Geometry: final body of the model. Coordinates: model frame, mm. A direction names the side the tool comes from. Coordinates: 2 decimals unless noted, no trailing zeros. Loops run counter-clockwise (first coordinate to the right, second up) from the corner with the lowest first, then second, coordinate; pieces in that order, holes last. Notation, with made-up numbers: (71.25, -16.5) - (107.25, -16.5) arc R12 ccw to (107.25, -12.5) - close; hole circle Ø7 at (61, -12). An arc over 180 degrees is marked (long way). Answer in a Markdown table with one row per item.
from build123d import *

# Parameters (mm, degrees)
ESQUISSE1_W           = 11.4
ESQUISSE1_H           = 11.4
BOSS_EXTRU_1_DEPTH    = 147.2
TROU_TARAUD_M41_D     = 3.3
TROU_TARAUD_M41_DEPTH = 11.5
TROU_TARAUD_M41_TIP   = 0.991420021
TROU_TARAUD_M42_D     = 3.3
TROU_TARAUD_M42_DEPTH = 11.5
TROU_TARAUD_M42_TIP   = 0.991420021
D_GAGEMENT_M41_D      = 4.5


with BuildPart() as part:
    # Esquisse1 → Boss.-Extru.1 (new body)
    with BuildSketch(Plane(origin=(0, 0, 0), x_dir=(1, 0, 0), z_dir=(0, 1, 0))):
        Rectangle(ESQUISSE1_W, ESQUISSE1_H)
    extrude(amount=BOSS_EXTRU_1_DEPTH)

    # Trou taraudé M41
    with Locations(Plane(origin=(0, 147.2, 0), x_dir=(-1, 0, 0), z_dir=(0, 1, 0))):
        with Locations((0, 0)):
            Hole(TROU_TARAUD_M41_D / 2, depth=TROU_TARAUD_M41_DEPTH)
            with Locations((0, 0, -(TROU_TARAUD_M41_DEPTH + TROU_TARAUD_M41_TIP / 2))):  # 118° drill point
                Cone(0, TROU_TARAUD_M41_D / 2, TROU_TARAUD_M41_TIP, mode=Mode.SUBTRACT)

    # Trou taraudé M42
    with Locations(Plane.XZ):
        with Locations((0, 0)):
            Hole(TROU_TARAUD_M42_D / 2, depth=TROU_TARAUD_M42_DEPTH)
            with Locations((0, 0, -(TROU_TARAUD_M42_DEPTH + TROU_TARAUD_M42_TIP / 2))):  # 118° drill point
                Cone(0, TROU_TARAUD_M42_D / 2, TROU_TARAUD_M42_TIP, mode=Mode.SUBTRACT)

    # Dégagement M41 (through all)
    with Locations(Plane.XY.offset(5.7)):
        with Locations((0, 128.6), (0, 73.6), (0, 18.6)):
            Hole(D_GAGEMENT_M41_D / 2)


solid = part.part
(1) Cut plane A-A on y = 18.6. Output: boundary loops of the cut face in (x, z).
Verdict:
| item | result |
|---|---|
| outline | (-5.7, -5.7) - (-2.25, -5.7) - (-2.25, 5.7) - (-5.7, 5.7) - close; (2.25, -5.7) - (5.7, -5.7) - (5.7, 5.7) - (2.25, 5.7) - close |
(2) Pull-direction query (Y, two-part tool) for faces 4 (the face through (0.488, 71.404, -0.08)), 5 (the face through (-1.3, 0, -1.3)), 6 (the face through (-3, 73, -5.7)); classes: pulls with the +Y half, pulls with the -Y half, needs draft (parallel to the pull), parting line crosses it, or undercut.
Verdict:
| item | result |
|---|---|
| face 4 | undercut |
| face 5 | pulls with the -Y half |
| face 6 | needs draft |
(3) Access query for faces 1 (the face through (-1.216, 141.37, 1.115)), 2 (the face through (5.7, 73, 0)), 3 (the face through (1.216, 5.831, 1.115)). Directions: +Z, -Z, +X, -X, +Y, -Y. A direction counts if a zero-diameter tool reaches every point of the face in a straight line with its end or side. Return the directions, or none.
Verdict:
| item | result |
|---|---|
| face 1 | +Y |
| face 2 | +Z, -Z, +X, +Y, -Y |
| face 3 | -Y |
(4) Cut plane B-B on z = 4.5. Output: boundary loops of the cut face in (x, y).
Verdict:
| item | result |
|---|---|
| outline | (-5.7, 0) - (5.7, 0) - (5.7, 147.2) - (-5.7, 147.2) - close; hole circle Ø4.5 at (0, 18.6); hole circle Ø4.5 at (0, 73.6); hole circle Ø4.5 at (0, 128.6) |
(5) Ray query, probe 1 along Y at (x, z) = (0, 1.75); probe 2 along X at (y, z) = (128.6, -1.75); probe 3 along Z at (x, y) = (0, 142.75). Return the intervals inside material, ascending.
Verdict:
| item | result |
|---|---|
| probe 1 | y = 0 to 16.35, 20.85 to 71.35, 75.85 to 126.35, 130.85 to 147.2 |
| probe 2 | x = -5.7 to -2.25, 2.25 to 5.7 |
| probe 3 | z = -5.7 to -1.65, 1.65 to 5.7 |
(6) First-contact query: pin 1 Ø1.5 at (x, z) = (0, 4.5) entering from -Y; pin 2 Ø2 at (x, z) = (0, 0) entering from -Y; pin 3 Ø2 at (x, z) = (0.5, 0) entering from +Y. Flat tips, straight axial feed; report the tip coordinate or a pass-through.
Verdict:
| item | result |
|---|---|
| pin 1 | stops at y = 0 |
| pin 2 | stops at y = 11.89 |
| pin 3 | stops at y = 135.61 |
(7) Cut plane C-C on y = 137. Output: boundary loops of the cut face in (x, z).
Verdict:
| item | result |
|---|---|
| outline | (-5.7, -5.7) - (5.7, -5.7) - (5.7, 5.7) - (-5.7, 5.7) - close; hole circle Ø3.3 at (0, 0) |
